Here's how the part is built. I have some questions about the finished solid (model axes, mm). A direction names the side the tool comes from. Give positions to 0.01 mm unless a question says otherwise; leave off trailing zeros. Write each loop counter-clockwise with the first axis right and the second up, starting at its lowest first coordinate (ties: lowest second). Pieces come first, ordered by that corner, then holes. Notation, with made-up numbers: (7, 35.25) -> (27, 35.25) arc R12 cw to (27, 49.25) -> close; hole circle Ø2 at (4, 84.5). An arc over 180 degrees is marked (long way). Use one line per item in the form item = value.
Autodesk Inventor part; units mm, degrees
ref_plane "YZ Plane" through (0, 0, 0) normal (1, 0, 0) x (0, 1, 0)
ref_plane "XZ Plane" through (0, 0, 0) normal (0, 1, 0) x (-1, 0, 0)
ref_plane "XY Plane" through (0, 0, 0) normal (0, 0, 1) x (1, 0, 0)
sketch "草圖1" plane through (0, 0, 0) normal (0, 1, 0) x (-1, 0, 0)
  line L0 (0, 0) -> (40, 0)
  line L1 (40, 0) -> (40, -60)
  line L2 (30, -70) -> (10, -70)
  line L3 (0, -60) -> (0, 0)
  circle A0 centre (20, -50) radius 10
  arc A1 (30, -70) -> (40, -60) centre (30, -60) ccw
  arc A2 (0, -60) -> (10, -70) centre (10, -60) ccw
  line L4 (0, -10) -> (30, -10)
  line L5 (30, -10) -> (30, -30)
  line L6 (30, -30) -> (40, -30)
  point P0 (40, -70)
  point P1 (0, -70)
  point P2 (40, -10)
  point P3 (0, -30)
  dimension "d0" = 40
  dimension "d1" = 70
  dimension "d5" = 20
  dimension "d6" = 20
  dimension "d7" = 20
  dimension "d8" = 10
  dimension "d18" = 30
  dimension "d19" = 20
  dimension "d20" = 10
extrude "擠出1" add sketch "草圖1" along normal blind 40 contours L0 L1 L6 L5 L4 L3
extrude "擠出2" add sketch "草圖1" along normal blind 20
sketch "草圖3" plane through (0, 0, 0) normal (1, 0, 0) x (0, 0, -1)
  line L0 (10, 40) -> (30, 20)
  line L1 (10, 20) -> (10, 40)
  line L2 (30, 20) -> (10, 20)
  line L3 (10, 20) -> (10, 40)
  point P0 (0, 0)
extrude "擠出4" add sketch "草圖3" against normal blind 10
Q1. If we mould it in two halves opening along X, with no side actions, what happens to faces 6 (the face through (-20, 0, -35)), 7 (the face through (-19.7, 20, -39.6)), 8 (the face through (-3.01, 9.86, -67.15))? For each: +X half, -X half, draft (parallel to the pull), parting line (faces both ways), or undercut.
Result set:
face_6 = draft
face_7 = undercut
face_8 = +X half
Q2. I want a section at B-B, the plane y = 9. Write out the boundary of the cut face in (x, z).
Result set:
outline = (-40, -60) arc R10 ccw to (-30, -70) -> (-10, -70) arc R10 ccw to (0, -60) -> (0, 0) -> (-40, 0) -> close; hole circle Ø20 at (-20, -50)
Q3. I want a section at D-D, the plane z = -25. Write out the boundary of the cut face in (x, y), and give its area (3 significant figures).
Result set:
outline = (-40, 0) -> (0, 0) -> (0, 25) -> (-10, 25) -> (-10, 20) -> (-30, 20) -> (-30, 40) -> (-40, 40) -> close
area = 1,050 mm2
Q4. I want a section at A-A, the plane z = -50. Write out the boundary of the cut face in (x, y).
Result set:
outline = (-40, 0) -> (-30, 0) -> (-30, 20) -> (-40, 20) -> close; (-10, 0) -> (0, 0) -> (0, 20) -> (-10, 20) -> close
Q5. If I drill on line 1 along Z through (x, y) = (-20, 9.25); line 2 along X through (y, z) = (17.5, -52.5); line 3 along X through (y, z) = (11.5, -58), over which ranges is the centre line in solid material (lowest first)? Write a range as from..to.
Result set:
line_1 = -70..-60, -40..0
line_2 = -40..-29.68, -10.32..0
line_3 = -40..-26, -14..0
Q6. Which directions (+Z, -Z, +X, -X, +Y, -Y) give clear straight access to the entire face, cutting with the end or side of a thin tool? Please do faces 1 (the face through (-35, 30, -30)), 2 (the face through (0, 16, -23)), 3 (the face through (-37.15, 9.86, -66.99)), 4 (the face through (-5, 30, -20)), 5 (the face through (-30, 30, -20)).
Result set:
face_1 = -Z, +X, -X, +Y
face_2 = +Z, -Z, +X, +Y, -Y
face_3 = -Z, -X, +Y, -Y
face_4 = -Z, +X, +Y
face_5 = -Z, +Y
Q7. I want a section at C-C, the plane x = -20. Write out the boundary of the cut face in (y, z).
Result set:
outline = (0, -70) -> (20, -70) -> (20, -60) -> (0, -60) -> close; (0, -40) -> (20, -40) -> (20, -10) -> (40, -10) -> (40, 0) -> (0, 0) -> close
Q8. Will these pins go through, and if not, where does the flat tip stop? pin 1 Ø1 at (x, y) = (-6, 5.5) entering from -Z; pin 2 Ø3 at (x, y) = (-33, 28) entering from -Z; pin 3 Ø12 at (x, z) = (-24.5, -40.5) entering from +Y.
Result set:
pin_1 = -69.37
pin_2 = -30
pin_3 = 20
